from build123d import *

# Parameters (mm, degrees)
EXTRUDE_1_DEPTH     = 2
EXTRUDE_START       = -2
EXTRUDE_6_DEPTH     = 2
SKETCH_3_R          = 1.45
CUT_EXTRUDE_1_DEPTH = 2
EXTRUDE_START_2     = -20
EXTRUDE_7_DEPTH     = 20
SKETCH_6_R          = 1.45
CUT_EXTRUDE_2_DEPTH = 20


# Read off the part's stored shape, not the designer's step: the extrude step
with BuildPart() as part:
    # Sketch 1 → Extrude 1 (new body)
    with BuildSketch(Plane.XY):
        with BuildLine():
            ThreePointArc((34.999399669, -35.707730574), (0, -50), (-34.999399669, -35.707730574))
            ThreePointArc((-34.999399669, -35.707730574), (-40.655970089, -35.764397047), (-40.599303617, -41.420967466))
            ThreePointArc((-40.599303617, -41.420967466), (0, -58), (40.599303617, -41.420967466))
            ThreePointArc((40.599303617, -41.420967466), (40.655970089, -35.764397047), (34.999399669, -35.707730574))
        make_face()
    extrude(amount=EXTRUDE_1_DEPTH)

    # Sketch 2 → Extrude 6 (add)
    with BuildSketch(Plane.XY.offset(2).offset(EXTRUDE_START)):
        with BuildLine():
            add(Edge.make_bspline(
                [(-34.999399669, -35.707730574), (-31.293036679, -34.051470167), (-32.304776642, -38.162827543)],
                knots=[0, 0, 0, 1, 1, 1], degree=2))
            ThreePointArc((-34.999399669, -35.707730574), (-33.674469744, -36.959844257), (-32.304776642, -38.162827543))
        make_face()
        with BuildLine():
            add(Edge.make_bspline(
                [(-29.427336681, -40.423159895), (-26.001624486, -38.244898865), (-26.403964274, -42.459753539)],
                knots=[0, 0, 0, 1, 1, 1], degree=2))
            ThreePointArc((-29.427336681, -40.423159895), (-27.934216832, -41.469018918), (-26.403964274, -42.459753539))
        make_face()
        with BuildLine():
            add(Edge.make_bspline(
                [(-23.228081101, -44.277039743), (-20.15603281, -41.623203943), (-19.940397248, -45.851723605)],
                knots=[0, 0, 0, 1, 1, 1], degree=2))
            ThreePointArc((-23.228081101, -44.277039743), (-21.598594585, -45.094353437), (-19.940397248, -45.851723605))
        make_face()
        with BuildLine():
            add(Edge.make_bspline(
                [(-16.5337593, -47.18723136), (-13.880850288, -44.114382693), (-13.051835275, -48.266443788)],
                knots=[0, 0, 0, 1, 1, 1], degree=2))
            ThreePointArc((-16.5337593, -47.18723136), (-14.802635794, -47.758580104), (-13.051835275, -48.266443788))
        make_face()
        with BuildLine():
            add(Edge.make_bspline(
                [(-9.487049125, -49.091709065), (-7.309821542, -45.665339966), (-5.885096092, -49.65244852)],
                knots=[0, 0, 0, 1, 1, 1], degree=2))
            ThreePointArc((-9.487049125, -49.091709065), (-7.69118452, -49.404915552), (-5.885096092, -49.65244852))
        make_face()
        with BuildLine():
            add(Edge.make_bspline(
                [(-2.238138968, -49.949882222), (-0.58299664, -46.243019798), (1.407073696, -49.980197515)],
                knots=[0, 0, 0, 1, 1, 1], degree=2))
            ThreePointArc((-2.238138968, -49.949882222), (-0.415809002, -49.998270999), (1.407073696, -49.980197515))
        make_face()
        with BuildLine():
            add(Edge.make_bspline(
                [(5.058473235, -49.743460359), (6.156253823, -45.835109949), (8.669254151, -49.242705373)],
                knots=[0, 0, 0, 1, 1, 1], degree=2))
            ThreePointArc((5.058473235, -49.743460359), (6.868428764, -49.526000104), (8.669254151, -49.242705373))
        make_face()
        with BuildLine():
            add(Edge.make_bspline(
                [(31.66559238, -38.694835046), (30.424637319, -34.829559417), (34.400675338, -36.284894051)],
                knots=[0, 0, 0, 1, 1, 1], degree=2))
            ThreePointArc((31.66559238, -38.694835046), (33.055103788, -37.514798594), (34.400675338, -36.284894051))
        make_face()
        with BuildLine():
            add(Edge.make_bspline(
                [(25.69413065, -42.893025659), (25.029188635, -38.888256343), (28.750957058, -40.906997791)],
                knots=[0, 0, 0, 1, 1, 1], degree=2))
            ThreePointArc((25.69413065, -42.893025659), (27.240649231, -41.927878905), (28.750957058, -40.906997791))
        make_face()
        with BuildLine():
            add(Edge.make_bspline(
                [(19.175043133, -46.177025899), (19.100286249, -42.118117602), (22.488462044, -44.657239893)],
                knots=[0, 0, 0, 1, 1, 1], degree=2))
            ThreePointArc((19.175043133, -46.177025899), (20.84560753, -45.44733927), (22.488462044, -44.657239893))
        make_face()
        with BuildLine():
            add(Edge.make_bspline(
                [(12.247272863, -48.476843002), (12.764294423, -44.450304307), (15.746664505, -47.455690459)],
                knots=[0, 0, 0, 1, 1, 1], degree=2))
            ThreePointArc((12.247272863, -48.476843002), (14.006277895, -47.998168502), (15.746664505, -47.455690459))
        make_face()
    extrude(amount=EXTRUDE_6_DEPTH)

    # Sketch 3 → Cut-Extrude 1 (cut)
    with BuildSketch(Plane.XY.offset(2)):
        with Locations((-37.799351643, -38.56434902)):
            Circle(SKETCH_3_R)
        with Locations((0, -53.900429622)):
            Circle(SKETCH_3_R)
        with Locations((37.799351643, -38.56434902)):
            Circle(SKETCH_3_R)
    extrude(amount=-CUT_EXTRUDE_1_DEPTH, mode=Mode.SUBTRACT)

    # Extrude 7 outline → Extrude 7 (add)
    with BuildSketch(Plane.XY.offset(2).offset(EXTRUDE_START_2)):
        with BuildLine():
            ThreePointArc((13.738692935, -56.349341757), (-0.341019933, -57.998997452), (-14.400360847, -56.183890996))
            Line((-14.400360847, -56.183890996), (-8, -60.499906827))
            Line((-8, -60.499906827), (8, -60.499906827))
            Line((8, -60.499906827), (13.738692935, -56.349341757))
        make_face()
    extrude(amount=EXTRUDE_7_DEPTH)

    # Sketch 6 → Cut-Extrude 2 (cut)
    with BuildSketch(Plane.XZ.offset(60.499906827)):
        with Locations(Location((-4.94974747, -5.05, 0), (0, 0, 270))):
            Circle(SKETCH_6_R)
        with Locations(Location((-4.94974747, -14.94949494, 0), (0, 0, 270))):
            Circle(SKETCH_6_R)
        with Locations(Location((4.94974747, -14.94949494, 0), (0, 0, 270))):
            Circle(SKETCH_6_R)
        with Locations(Location((4.94974747, -5.05, 0), (0, 0, 270))):
            Circle(SKETCH_6_R)
    extrude(amount=-CUT_EXTRUDE_2_DEPTH, mode=Mode.SUBTRACT)


solid = part.part
The model under review builds one solid part; all positions refer to its coordinate system, in mm. A direction names the side the tool comes from. Round coordinates to 2 decimals unless told otherwise and drop trailing zeros. Write each loop counter-clockwise with the first axis right and the second up, starting at its lowest first coordinate (ties: lowest second). Pieces come first, ordered by that corner, then holes. Notation, with made-up numbers: (-38.75, 62.25) -> (-11.75, 62.25) arc R24 ccw to (-11.75, 87.25) -> close; hole circle Ø5 at (45, 84). An arc over 180 degrees is marked (long way). Answer as a JSON object with one key per item and string values.
1. We need section B-B on x = 24.5. State the section outline as (y, z) points.
Results found:
{"outline": "(-52.57, 0) -> (-43.59, 0) -> (-43.59, 2) -> (-52.57, 2) -> close"}
2. Clearance check with flat-ended pins moving along their axes: pin 1 (2.5 mm diameter, centred on x = 4.95, z = -5.05, fed in from -Y); pin 2 (3.5 mm diameter, centred on x = 0, y = -53.9, fed in from -Z); pin 3 (5 mm diameter, centred on x = 3, z = -0.5, fed in from +Y); pin 4 (4.5 mm diameter, centred on x = 4.95, z = -14.95, fed in from +Y). State where each tip first meets the part, or that it passes through.
Results found:
{"pin 1": "passes through", "pin 2": "stops at z = 0", "pin 3": "stops at y = -48.67", "pin 4": "stops at y = -57.55"}
3. We need section A-A on z = -5.05. State the section outline as (x, y) points, and give its area (3 significant figures).
Results found:
{"outline": "(-14.4, -56.18) -> (-8, -60.5) -> (-6.4, -60.5) -> (-6.4, -57.65) arc R58 cw to start; (-3.5, -60.5) -> (3.5, -60.5) -> (3.5, -57.89) arc R58 cw to (-3.5, -57.89) -> close; (6.4, -60.5) -> (8, -60.5) -> (13.74, -56.35) arc R58 cw to (6.4, -57.65) -> close", "area": "45.0 mm^2"}
4. Machinability: for faces 1 (the face through (6.387, -59.093, -4.861)), 2 (the face through (-18.23, -46.56, 0.99)), 3 (the face through (0, -58, -9)), which of the approach directions +Z, -Z, +X, -X, +Y, -Y give a long, thin tool a straight path to every point of the face, cutting with its end or side? Answer none if there is none.
Results found:
{"face 1": "+Y, -Y", "face 2": "+Z, -Z, +Y", "face 3": "-Z, +Y"}
5. The part is to be moulded in two halves that separate along Z. For faces 4 (the face through (6.387, -59.093, -14.761)), 5 (the face through (24.13, -43.79, 0.99)), 6 (the face through (0, -50, 0)), say which applies: pulls with the +Z half, pulls with the -Z half, needs draft (parallel to the pull), parting line crosses it, or undercut.
Results found:
{"face 4": "undercut", "face 5": "needs draft", "face 6": "pulls with the -Z half"}
6. To check wall thickness, follow line 1 along X through (y, z) = (-48.25, 1); line 2 along X through (y, z) = (-58.7, -5.05); line 3 along Z through (x, y) = (34, -45). State the ranges of each line that lie inside material, in increasing order.
Results found:
{"line 1": "x = -32.19 to -13.06, -8.87 to -6.55, -1.01 to 0.01, 5.69 to 7.81, 12.28 to 32.19", "line 2": "x = -10.67 to -6.4, -3.5 to 3.5, 6.4 to 10.49", "line 3": "z = 0 to 2"}
